Read the model definition and answer for the solid it produces. Units are mm, in the model's axes. A direction names the side the tool comes from. Coordinates: 2 decimals unless noted, no trailing zeros. Order: outer loops, then holes, each group sorted by start corner. A loop starts at its lowest first (then second) coordinate and runs counter-clockwise, first axis right, second up. Notation, with made-up numbers: (13.25, 46.25) -> (37.25, 46.25) arc R20 cw to (37.25, 82.25) -> close; hole circle Ø5 at (1.5, -22.5). An arc over 180 degrees is marked (long way). Use CSV: the item, a comma, the result in double quotes.
```python
from build123d import *

# Parameters (mm, degrees)
SKETCH1_R           = 5
BOSS_EXTRUDE1_DEPTH = 5
BOSS_EXTRUDE2_DEPTH = 10
SKETCH3_W           = 12
SKETCH3_H           = 12
BOSS_EXTRUDE3_DEPTH = 22
SKETCH4_W           = 35
SKETCH4_H           = 35
BOSS_EXTRUDE4_DEPTH = 1
FILLET1_R           = 10
FILLET4_R           = 5


with BuildPart() as part:
    # Sketch1 → Boss-Extrude1 (new body)
    with BuildSketch(Plane(origin=(0, 0, 0), x_dir=(1, 0, 0), z_dir=(0, 1, 0))):
        Polygon((0, 0), (0, 35), (35, 35), (35, 0), (35, -14), (21, -14), (21, 0), align=None)
        with Locations(Location((28, -7, 0), (0, 0, 270))):
            Circle(SKETCH1_R, mode=Mode.SUBTRACT)
        with BuildLine():
            Line((5.77728435, 32.399644503), (19.919419974, 18.257508879))
            ThreePointArc((19.919419974, 18.257508879), (19.829534471, 14.632089471), (16.21302376, 14.901525103))
            Line((16.21302376, 14.901525103), (2.070888136, 29.043660727))
            ThreePointArc((2.070888136, 29.043660727), (2.160773638, 32.669080135), (5.77728435, 32.399644503))
        make_face(mode=Mode.SUBTRACT)
    extrude(amount=BOSS_EXTRUDE1_DEPTH)

    # Sketch2 → Boss-Extrude2 (add)
    with BuildSketch(Plane.XZ):
        Polygon((30, -5), (20, -5), (20, 0), (35, 0), (35, -15), (30, -15), align=None)
    extrude(amount=BOSS_EXTRUDE2_DEPTH)

    # Sketch3 → Boss-Extrude3 (add)
    with BuildSketch(Plane(origin=(0, 5, 0), x_dir=(1, 0, 0), z_dir=(0, 1, 0))):
        with Locations((6, 6)):
            Rectangle(SKETCH3_W, SKETCH3_H)
    extrude(amount=BOSS_EXTRUDE3_DEPTH)

    # Sketch4 → Boss-Extrude4 (add)
    with BuildSketch(Plane(origin=(0, 27, 0), x_dir=(1, 0, 0), z_dir=(0, 1, 0))):
        with Locations((17.5, 17.5)):
            Rectangle(SKETCH4_W, SKETCH4_H)
    extrude(amount=BOSS_EXTRUDE4_DEPTH)

    # Fillet1
    # the kernel refuses this fillet: 10 mm, written as the material it adds along each edge
    with BuildSketch(Plane(origin=(21, 0, 0), x_dir=(0, 0, 1), z_dir=(0, 1, 0))) as fillet1_piece_1:
        with BuildLine():
            CenterArc((FILLET1_R, -FILLET1_R), FILLET1_R, 90, 90)
            Line((0, -FILLET1_R), (0, 0))
            Line((0, 0), (FILLET1_R, 0))
        make_face()
    extrude(amount=5)

    # Fillet4
    fillet4_edges = [part.edges().sort_by_distance(p)[0] for p in [
        (35, 2.5, 14),
        (21, 2.5, 14),
    ]]
    fillet(fillet4_edges, radius=FILLET4_R)


solid = part.part
```
Item 1: Find section C-C, the plane z = 7. Give the vertices of the cut face in (x, y), then the cut area to 3 significant figures.
Return value:
outline,"(20.54, 0) -> (23, 0) -> (23, 5) -> (20.54, 5) -> close; (33, 0) -> (35, 0) -> (35, 5) -> (33, 5) -> close"
area,"22.3 mm^2"
Item 2: Straight lines are drawn through the part: line 1 along Y through (x, z) = (27.5, -25.5); line 2 along Y through (x, z) = (30, -4); line 3 along Z through (x, y) = (2, 16). For each, find the intervals that lie inside material, in ascending order.
Return value:
line 1,"y = 0 to 5, 27 to 28"
line 2,"y = -10 to 5, 27 to 28"
line 3,"z = -12 to 0"
Item 3: Each of these flat-tipped pins is pushed along its axis until it touches: P1, Ø8, axis at x = 25, y = -6, coming from the -Z side; P2, Ø11, axis at y = -7, z = -12, coming from the -X side; P3, Ø3.5, axis at x = 8.5, y = 13, coming from the -Z side. Where does it stop, or does it pass through?
Return value:
P1,"stops at z = -5"
P2,"stops at x = 30"
P3,"stops at z = -12"
Item 4: The mould has two halves that part along Z. Classify faces 1 (the cylindrical face through (23.564, 2.465, 9.307)), 2 (the cylindrical face through (33, 3, 13)), 3 (the flat face through (30, -5, -10)): +Z half, -Z half, draft (parallel to the pull), parting line (faces both ways), or undercut.
Return value:
face 1,"undercut"
face 2,"+Z half"
face 3,"draft"
Item 5: Find section B-B, the plane z = -19. Give the vertices of the cut face in (x, y), then the cut area to 3 significant figures.
Return value:
outline,"(0, 0) -> (12.11, 0) -> (12.11, 5) -> (0, 5) -> close; (0, 27) -> (35, 27) -> (35, 28) -> (0, 28) -> close; (19.18, 0) -> (35, 0) -> (35, 5) -> (19.18, 5) -> close"
area,"175 mm^2"
Item 6: Find section D-D, the plane y = -7. Give the vertices of the cut face in (x, z), then the cut area to 3 significant figures.
Return value:
outline,"(20, -5) -> (30, -5) -> (30, -15) -> (35, -15) -> (35, 0) -> (20, 0) -> close"
area,"125 mm^2"
Item 7: Find section A-A, the plane x = 28. Give the vertices of the cut face in (y, z), then the cut area to 3 significant figures.
Return value:
outline,"(-10, -5) -> (0, -5) -> (0, -35) -> (5, -35) -> (5, 2) -> (0, 2) -> (0, 0) -> (-10, 0) -> close; (0, 12) -> (5, 12) -> (5, 14) -> (0, 14) -> close; (27, -35) -> (28, -35) -> (28, 0) -> (27, 0) -> close"
area,"280 mm^2"
Item 8: A tool of negligible diameter and unlimited length cuts with its end or side. For faces 4 (the flat face through (6, 16, -12)), 5 (the flat face through (12.749, 2.465, -25.428)), 6 (the flat face through (17, 27, -18)), 7 (the flat face through (12, 16, -6)), from which of +Z, -Z, +X, -X, +Y, -Y can it reach the whole face along a straight path? Write none if from no direction.
Return value:
face 4,"-Z, +X, -X"
face 5,"-Y"
face 6,"-Z, +X"
face 7,"+Z, -Z, +X"
